Design review of the part built by this model. Coordinates are the model's own, in mm. A direction names the side the tool comes from. Round coordinates to 2 decimals unless told otherwise and drop trailing zeros. Write each loop counter-clockwise with the first axis right and the second up, starting at its lowest first coordinate (ties: lowest second). Pieces come first, ordered by that corner, then holes. Notation, with made-up numbers: (-22, 20.25) -> (21, 20.25) arc R25 ccw to (21, 33.25) -> close; hole circle Ø7 at (86, -40). An arc over 180 degrees is marked (long way). One line per question, with ' | ' between items. Start each with the question number.
1) Consider section C-C (y = 0.85). Count the separate pieces of the cut face and the enclosed holes in it, then the cut area to 3 significant figures.
2) For probe 1 along X at (y, z) = (2.65, 22); probe 2 along X at (y, z) = (2.95, 34); probe 3 along Z at (x, y) = (45.78, 3.7) (3 decimals), list the stretches that pass through material, from the lowest coordinate up.
3) Consider section B-B (x = 57.55). Give the boundary of the cut face in (y, z), then the cut area to 3 significant figures.
4) For faces 1 (the flat face through (57, 2, 66)), 2 (the flat face through (27, 2, 33.5)), list the 3-axis set-ups (+Z, -Z, +X, -X, +Y, -Y) from which the entire face can be reached by the end or side of a thin tool; tool diameter is ignored.
5) Consider section D-D (x = 37.55). Give the boundary of the cut face in (y, z).
6) Mouldability with a two-part tool opening along X and no side actions: class faces 3 (the flat face through (27, 2, 16.5)), 4 (the flat face through (57, 2, 0)) as +X half, -X half, draft (parallel to the pull), parting line (faces both ways), or undercut.
7) Insertion check: pin 1 Ø0.8 at (x, z) = (29.5, 13.5) entering from -Y. The pin has a flat end and moves straight along its axis. Give the tip position at first contact, or say it passes through.
8) Consider section A-A (x = 97). Give the boundary of the cut face in (y, z), then the cut area to 3 significant figures.
```python
from build123d import *

# Parameters (mm, degrees)
SKETCH_1_W             = 115.1
SKETCH_1_H             = 66
EXTRUDE_1_DEPTH        = 5
SKETCH_1_3_W           = 1
SKETCH_1_3_H           = 1
SKETCH_1_3_H_2         = 1.5
SKETCH_1_3_W_2         = 1.2
SKETCH_1_3_H_3         = 1.2
CUT_EXTRUDE_1_DEPTH    = 133.774282148
PATTERN_LINEAR_1_COUNT = 2
PATTERN_LINEAR_1_PITCH = 75
SKETCH_1_4_R           = 0.75
SKETCH_1_4_W           = 18.5
SKETCH_1_4_H           = 3
CUT_EXTRUDE_2_DEPTH    = 133.774282148
SKETCH_2_R             = 4
CUT_EXTRUDE_3_DEPTH    = 133.774282148
SKETCH_5_R             = 0.75
CUT_EXTRUDE_4_DEPTH    = 3
SKETCH_6_R             = 0.75
CUT_EXTRUDE_5_DEPTH    = 4
CUT_EXTRUDE_START      = -111.1
SKETCH_6_4_R           = 0.75
CUT_EXTRUDE_6_DEPTH    = 4
SKETCH_7_R             = 0.75
CUT_EXTRUDE_7_DEPTH    = 4
CUT_EXTRUDE_START_2    = -62
SKETCH_7_2_R           = 0.75
CUT_EXTRUDE_8_DEPTH    = 4


with BuildPart() as part:
    # 草图1 → 凸台-拉伸1 (new body)
    with BuildSketch(Plane(origin=(0, 0, 0), x_dir=(1, 0, 0), z_dir=(0, 1, 0))):
        with Locations((57.55, -33)):
            Rectangle(SKETCH_1_W, SKETCH_1_H)
    extrude(amount=EXTRUDE_1_DEPTH)

    # 草图1<3> → 切除-拉伸1 (cut, through all)
    with BuildSketch(Plane(origin=(0, 0, 0), x_dir=(1, 0, 0), z_dir=(0, 1, 0))):
        Polygon((25, -33.5), (15, -33.5), (15, -34.5), (15, -39.7), (25, -39.7), (25, -34.5), align=None)
        with Locations((25.5, -34)):
            Rectangle(SKETCH_1_3_W, SKETCH_1_3_H)
        with Locations((14.5, -34)):
            Rectangle(SKETCH_1_3_W, SKETCH_1_3_H)
        Polygon((11.5, -16.5), (11.5, -18.7), (11.5, -20.2), (11.5, -29.6), (11.5, -31.1), (11.5, -33.5), (14, -33.5), (15, -33.5), (25, -33.5), (26, -33.5), (28.3, -33.5), (28.3, -31.1), (28.3, -29.9), (29.5, -29.9), (31.5, -29.9), (31.5, -19.9), (29.6, -19.9), (28.4, -19.9), (25, -19.9), (25, -16.5), (25, -15.3), (25, -13.5), (15, -13.5), (15, -15.3), (15, -16.5), (13.8, -16.5), align=None)
        with Locations((11, -30.35)):
            Rectangle(SKETCH_1_3_W, SKETCH_1_3_H_2)
        with Locations((11, -19.45)):
            Rectangle(SKETCH_1_3_W, SKETCH_1_3_H_2)
        with Locations((25.6, -15.9)):
            Rectangle(SKETCH_1_3_W_2, SKETCH_1_3_H_3)
        Polygon((26.2, -16.5), (25, -16.5), (25, -19.9), (28.4, -19.9), (28.4, -18.7), (28.4, -16.5), align=None)
        with Locations((29, -19.3)):
            Rectangle(SKETCH_1_3_W_2, SKETCH_1_3_H_3)
        with Locations((28.9, -30.5)):
            Rectangle(SKETCH_1_3_W_2, SKETCH_1_3_H_3)
        with Locations((14.4, -15.9)):
            Rectangle(SKETCH_1_3_W_2, SKETCH_1_3_H_3)
    cut_extrude_1 = extrude(amount=CUT_EXTRUDE_1_DEPTH, mode=Mode.SUBTRACT)

    # 阵列(线性)1: 切除-拉伸1 ×2
    with Locations(*[(i * PATTERN_LINEAR_1_PITCH, 0, 0) for i in range(1, PATTERN_LINEAR_1_COUNT)]):
        add(cut_extrude_1, mode=Mode.SUBTRACT)

    # 草图1<4> → 切除-拉伸2 (cut, through all)
    with BuildSketch(Plane(origin=(0, 0, 0), x_dir=(1, 0, 0), z_dir=(0, 1, 0))):
        with Locations(Location((45.78, -15, 0), (0, 0, 270))):
            Circle(SKETCH_1_4_R)
        with Locations(Location((69.32, -15, 0), (0, 0, 270))):
            Circle(SKETCH_1_4_R)
        with Locations(Location((45.78, -38.545, 0), (0, 0, 270))):
            Circle(SKETCH_1_4_R)
        with Locations(Location((69.32, -38.545, 0), (0, 0, 270))):
            Circle(SKETCH_1_4_R)
        with Locations((57.55, -15)):
            Rectangle(SKETCH_1_4_W, SKETCH_1_4_H)
    extrude(amount=CUT_EXTRUDE_2_DEPTH, mode=Mode.SUBTRACT)

    # 草图2 → 切除-拉伸3 (cut, through all)
    with BuildSketch(Plane(origin=(0, 5, 0), x_dir=(1, 0, 0), z_dir=(0, 1, 0))):
        with Locations(Location((37.55, -49.474447741, 0), (0, 0, 270))):
            Circle(SKETCH_2_R)
        with Locations(Location((57.55, -49.474447741, 0), (0, 0, 270))):
            Circle(SKETCH_2_R)
        with Locations(Location((77.55, -49.474447741, 0), (0, 0, 270))):
            Circle(SKETCH_2_R)
    extrude(amount=-CUT_EXTRUDE_3_DEPTH, mode=Mode.SUBTRACT)

    # 草图5 → 切除-拉伸4 (cut)
    with BuildSketch(Plane.XZ):
        with Locations(Location((104.5, 35.5, 0), (0, 0, 270))):
            Circle(SKETCH_5_R)
        with Locations(Location((86.5, 13.5, 0), (0, 0, 270))):
            Circle(SKETCH_5_R)
        with Locations(Location((104.5, 13.5, 0), (0, 0, 270))):
            Circle(SKETCH_5_R)
        with Locations(Location((86.5, 35.5, 0), (0, 0, 270))):
            Circle(SKETCH_5_R)
        with Locations(Location((11.5, 35.5, 0), (0, 0, 270))):
            Circle(SKETCH_5_R)
        with Locations(Location((11.5, 13.5, 0), (0, 0, 270))):
            Circle(SKETCH_5_R)
        with Locations(Location((29.5, 13.5, 0), (0, 0, 270))):
            Circle(SKETCH_5_R)
        with Locations(Location((29.5, 35.5, 0), (0, 0, 270))):
            Circle(SKETCH_5_R)
        with Locations(Location((47.05, 48.924447741, 0), (0, 0, 270))):
            Circle(SKETCH_5_R)
        with Locations(Location((68.05, 48.924447741, 0), (0, 0, 270))):
            Circle(SKETCH_5_R)
    extrude(amount=-CUT_EXTRUDE_4_DEPTH, mode=Mode.SUBTRACT)

    # 草图6 → 切除-拉伸5 (cut)
    with BuildSketch(Plane.ZY):
        with Locations((15, 2.5)):
            Circle(SKETCH_6_R)
        with Locations((51, 2.5)):
            Circle(SKETCH_6_R)
    extrude(amount=-CUT_EXTRUDE_5_DEPTH, mode=Mode.SUBTRACT)

    # 草图6<4> → 切除-拉伸6 (cut)
    with BuildSketch(Plane.ZY.offset(CUT_EXTRUDE_START)):
        with Locations((15, 2.5)):
            Circle(SKETCH_6_4_R)
        with Locations((51, 2.5)):
            Circle(SKETCH_6_4_R)
    extrude(amount=-CUT_EXTRUDE_6_DEPTH, mode=Mode.SUBTRACT)

    # 草图7 → 切除-拉伸7 (cut)
    with BuildSketch(Plane.XY.offset(66)):
        with Locations((95.1, 2.5)):
            Circle(SKETCH_7_R)
        with Locations((20, 2.5)):
            Circle(SKETCH_7_R)
    extrude(amount=-CUT_EXTRUDE_7_DEPTH, mode=Mode.SUBTRACT)

    # 草图7<2> → 切除-拉伸8 (cut)
    with BuildSketch(Plane.XY.offset(66).offset(CUT_EXTRUDE_START_2)):
        with Locations((95.1, 2.5)):
            Circle(SKETCH_7_2_R)
        with Locations((20, 2.5)):
            Circle(SKETCH_7_2_R)
    extrude(amount=-CUT_EXTRUDE_8_DEPTH, mode=Mode.SUBTRACT)


solid = part.part
```
From the geometry:
1) separate pieces: 1 | enclosed holes: 20 | area: 6,520 mm2
2) probe 1: x = 0 to 11.5, 31.5 to 86.5, 106.5 to 115.1 | probe 2: x = 0 to 14, 26 to 89, 101 to 115.1 | probe 3: z = 0 to 14.25, 15.75 to 37.795, 39.295 to 66
3) outline: (0, 0) -> (5, 0) -> (5, 13.5) -> (0, 13.5) -> close; (0, 16.5) -> (5, 16.5) -> (5, 45.47) -> (0, 45.47) -> close; (0, 53.47) -> (5, 53.47) -> (5, 66) -> (0, 66) -> close | area: 275 mm2
4) face 1: +Z, +X, -X, +Y, -Y | face 2: +Y, -Y
5) outline: (0, 0) -> (5, 0) -> (5, 45.47) -> (0, 45.47) -> close; (0, 53.47) -> (5, 53.47) -> (5, 66) -> (0, 66) -> close
6) face 3: undercut | face 4: draft
7) pin 1: stops at y = 3
8) outline: (0, 0) -> (5, 0) -> (5, 13.5) -> (0, 13.5) -> close; (0, 39.7) -> (5, 39.7) -> (5, 66) -> (0, 66) -> close | area: 199 mm2
